The listing builds one solid part. Answer for the finished solid, in the listing's coordinates (mm). Face numbers are marked on the shaded views. A direction names the side the tool comes from. Give positions to 0.01 mm unless a question says otherwise; leave off trailing zeros. Loops run counter-clockwise (first coordinate to the right, second up) from the corner with the lowest first, then second, coordinate; pieces in that order, holes last. Notation, with made-up numbers: (-27, 9.25) - (-12, 9.25) arc R19 cw to (-12, 34.25) - close; hole circle Ø9 at (-32.5, -8.75). An arc over 180 degrees is marked (long way). Write each question's results on one line, items separated by ' | '.
from build123d import *


with BuildPart() as part:
    # 스케치1 → 회전1 (revolve)
    with BuildSketch(Plane(origin=(0, 0, 0), x_dir=(0, 0, -1), z_dir=(1, 0, 0))):
        with BuildLine():
            Line((12, 11.85), (-12, 11.85))
            Line((-12, 11.85), (-12, 10.9))
            Line((-12, 10.9), (-15, 10.9))
            Line((-15, 10.9), (-15, 10))
            Line((-15, 10), (-10, 10))
            ThreePointArc((-10, 10), (-9.688420677, 9.270526441), (-9.5, 8.5))
            Line((-9.5, 8.5), (-7.5, 8.5))
            Line((-7.5, 8.5), (-6.817399349, 10.732369836))
            Line((-6.817399349, 10.732369836), (6.817399349, 10.732369836))
            Line((6.817399349, 10.732369836), (7.5, 8.5))
            Line((7.5, 8.5), (9.5, 8.5))
            ThreePointArc((9.5, 8.5), (9.688420677, 9.270526441), (10, 10))
            Line((10, 10), (15, 10))
            Line((15, 10), (15, 10.9))
            Line((15, 10.9), (12, 10.9))
            Line((12, 10.9), (12, 11.85))
        make_face()
    revolve(axis=Axis((0, 0, 0), (0, 0, 1)))


solid = part.part
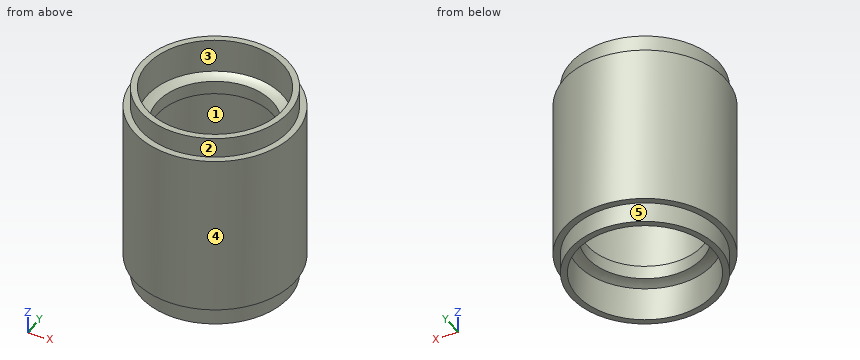
Item 1: For a pull along Y with two mould halves and no side action, classify the marked faces 1 and 2 as released by +Y, released by -Y, zero draft, split by the parting line, or undercut.
Values found:
face 1: undercut | face 2: split by the parting line
Item 2: A cutting plane is placed at C-C, the plane z = -1. Determine the outline of the cut face in (x, y).
Values found:
outline: circle Ø23.7 at (0, 0); hole circle Ø21.46 at (0, 0)
Item 3: Flat-ended cylindrical pins translate along their axes: P1, Ø1.5, axis at x = -8.5, y = 1, coming from the +Z side; P2, Ø6, axis at x = -8.5, z = -9, coming from the -Y side; P3, Ø8, axis at y = 1.5, z = -2, coming from the -X side; P4, Ø1.5, axis at y = 6.5, z = 7.5, coming from the -X side. Find the tip coordinate at first contact, or state that the pin passes through.
Values found:
P1: stops at z = 9.7 | P2: stops at y = -10.5 | P3: stops at x = -11.85 | P4: stops at x = -10.36
Item 4: Find the intervals of material crossed by line 1 along Y through (x, z) = (-5, 2.5); line 2 along Y through (x, z) = (0, 8.55); line 3 along X through (y, z) = (0, -11.7), in increasing order. Write a range as [from, to].
Values found:
line 1: y = [-10.74, -9.5], [9.5, 10.74] | line 2: y = [-11.85, -8.5], [8.5, 11.85] | line 3: x = [-11.85, -10], [10, 11.85]
Item 5: For the marked faces 3, 4 and 5, determine the directions among +Z, -Z, +X, -X, +Y, -Y from which every point of the face is accessible in a straight line to the end or side of a thin tool.
Values found:
face 3: +Z | face 4: +Z, -Z | face 5: -Z
